Geometry check sheet. Reference: the model listing, model coordinates, mm. A direction names the side the tool comes from. Give positions to 0.01 mm unless a question says otherwise; leave off trailing zeros. Order: outer loops, then holes, each group sorted by start corner. A loop starts at its lowest first (then second) coordinate and runs counter-clockwise, first axis right, second up.
```python
from build123d import *

# Parameters (mm, degrees)
SKETCH1_W            = 100
SKETCH1_H            = 85
SKETCH1_W_2          = 80
SKETCH1_H_2          = 65
BOSS_EXTRUDE1_DEPTH  = 40
SKETCH14_W           = 5
SKETCH14_H           = 5
CUT_EXTRUDE11_DEPTH  = 10
CUT_EXTRUDE16_REACH  = 117.785
SKETCH24_W           = 22
SKETCH24_H           = 22
BOSS_EXTRUDE13_DEPTH = 6
CUT_EXTRUDE17_REACH  = 108.419
SKETCH32_W           = 22
SKETCH32_H           = 22
BOSS_EXTRUDE17_DEPTH = 6
SKETCH33_W           = 5
SKETCH33_H           = 5
CUT_EXTRUDE18_DEPTH  = 10
SKETCH36_W           = 22
SKETCH36_H           = 22
BOSS_EXTRUDE19_DEPTH = 5


with BuildPart() as part:
    # Sketch1 → Boss-Extrude1 (new body)
    with BuildSketch(Plane(origin=(0, 0, 0), x_dir=(0, 1, 0), z_dir=(0, 0, 1))):
        Rectangle(SKETCH1_W, SKETCH1_H)
        Rectangle(SKETCH1_W_2, SKETCH1_H_2, mode=Mode.SUBTRACT)
    extrude(amount=BOSS_EXTRUDE1_DEPTH)

    # Sketch14 → Cut-Extrude11 (cut)
    with BuildSketch(Plane.XY.offset(40)):
        with Locations((-37.671132401, 44.6965107)):
            Rectangle(SKETCH14_W, SKETCH14_H)
        with Locations((-37.671132401, -44.6965107)):
            Rectangle(SKETCH14_W, SKETCH14_H)
        with Locations((37.671132401, 44.6965107)):
            Rectangle(SKETCH14_W, SKETCH14_H)
        with Locations((37.671132401, -44.6965107)):
            Rectangle(SKETCH14_W, SKETCH14_H)
        with Locations((0, 44.6965107)):
            Rectangle(SKETCH14_W, SKETCH14_H)
        with Locations((0, -44.6965107)):
            Rectangle(SKETCH14_W, SKETCH14_H)
        with Locations((-37.671132401, 0)):
            Rectangle(SKETCH14_W, SKETCH14_H)
    extrude(amount=-CUT_EXTRUDE11_DEPTH, mode=Mode.SUBTRACT)

    # Sketch22 → Cut-Extrude16 (cut, up to next)
    with BuildSketch(Plane(origin=(0, 50, 0), x_dir=(-1, 0, 0), z_dir=(0, 1, 0)), mode=Mode.PRIVATE) as cut_extrude16_sk1:
        with BuildLine():
            Line((-6, 9.521249719), (6, 9.521249719))
            ThreePointArc((6, 9.521249719), (10, 5.521249719), (6, 1.521249719))
            Line((6, 1.521249719), (-6, 1.521249719))
            ThreePointArc((-6, 1.521249719), (-10, 5.521249719), (-6, 9.521249719))
        make_face()
    cut_extrude16_tool1 = extrude(cut_extrude16_sk1.sketch, amount=-CUT_EXTRUDE16_REACH, mode=Mode.PRIVATE) & part.part
    add(cut_extrude16_tool1.solids().sort_by_distance((0, 50, 5.52125))[0], mode=Mode.SUBTRACT)

    # Sketch24 → Boss-Extrude13 (add)
    with BuildSketch(Plane.XY.offset(16)):
        with Locations((21.5, 2.716540801)):
            Rectangle(SKETCH24_W, SKETCH24_H)
    extrude(amount=BOSS_EXTRUDE13_DEPTH)

    # Sketch12 → Cut-Extrude17 (cut, up to next)
    with BuildSketch(Plane.YZ.offset(42.5), mode=Mode.PRIVATE) as cut_extrude17_sk1:
        with BuildLine():
            Line((-17.870386686, 34.517617013), (17.870386686, 34.517617013))
            ThreePointArc((17.870386686, 34.517617013), (19.229729644, 33.158274056), (17.870386686, 31.798931098))
            Line((17.870386686, 31.798931098), (-17.870386686, 31.798931098))
            ThreePointArc((-17.870386686, 31.798931098), (-19.229729644, 33.158274056), (-17.870386686, 34.517617013))
        make_face()
    cut_extrude17_tool1 = extrude(cut_extrude17_sk1.sketch, amount=-CUT_EXTRUDE17_REACH, mode=Mode.PRIVATE) & part.part
    # Sketch12 → Cut-Extrude17 (cut, up to next)
    with BuildSketch(Plane.YZ.offset(42.5), mode=Mode.PRIVATE) as cut_extrude17_sk2:
        with BuildLine():
            Line((-17.870386686, 29.316472465), (17.870386686, 29.316472465))
            ThreePointArc((17.870386686, 29.316472465), (19.31261641, 27.874242742), (17.870386686, 26.432013019))
            Line((17.870386686, 26.432013019), (-17.870386686, 26.432013019))
            ThreePointArc((-17.870386686, 26.432013019), (-19.31261641, 27.874242742), (-17.870386686, 29.316472465))
        make_face()
    cut_extrude17_tool2 = extrude(cut_extrude17_sk2.sketch, amount=-CUT_EXTRUDE17_REACH, mode=Mode.PRIVATE) & part.part
    add(cut_extrude17_tool1.solids().sort_by_distance((42.5, 0, 33.158274))[0], mode=Mode.SUBTRACT)
    add(cut_extrude17_tool2.solids().sort_by_distance((42.5, 0, 27.874243))[0], mode=Mode.SUBTRACT)

    # Sketch32 → Boss-Extrude17 (add)
    with BuildSketch(Plane.XY.offset(16)):
        with Locations((-2.810397874, 29)):
            Rectangle(SKETCH32_W, SKETCH32_H)
    extrude(amount=BOSS_EXTRUDE17_DEPTH)

    # Sketch33 → Cut-Extrude18 (cut)
    with BuildSketch(Plane(origin=(0, 0, 0), x_dir=(1, 0, 0), z_dir=(0, 0, -1))):
        with Locations((-37.671132401, 44.6965107)):
            Rectangle(SKETCH33_W, SKETCH33_H)
        with Locations((0, 44.6965107)):
            Rectangle(SKETCH33_W, SKETCH33_H)
        with Locations((37.671132401, 44.6965107)):
            Rectangle(SKETCH33_W, SKETCH33_H)
        with Locations((-37.671132401, 0)):
            Rectangle(SKETCH33_W, SKETCH33_H)
        with Locations((-37.671132401, -44.6965107)):
            Rectangle(SKETCH33_W, SKETCH33_H)
        with Locations((37.671132401, -44.6965107)):
            Rectangle(SKETCH33_W, SKETCH33_H)
    extrude(amount=-CUT_EXTRUDE18_DEPTH, mode=Mode.SUBTRACT)

    # Sketch36 → Boss-Extrude19 (add)
    with BuildSketch(Plane.XY.offset(23)):
        with Locations((-21.5, 3.296429393)):
            Rectangle(SKETCH36_W, SKETCH36_H)
    extrude(amount=BOSS_EXTRUDE19_DEPTH)


solid = part.part
```
Q1. Access from +Z, -Z, +X, -X, +Y, -Y to the whole of each face (thin tool, end or side, straight path). Record for faces 1 (the face through (-38, -45, 30)), 2 (the face through (38, 0, 34.518)), 3 (the face through (-40.171, 45, 5)), 4 (the face through (-13.81, 29, 19)).
Q2. Gauge pin test, flat ends, axial feed: P1, Ø2, axis at x = -24, y = 1, coming from the -Z side; P2, Ø6, axis at x = -30, y = 18.5, coming from the -Z side; P3, Ø11, axis at x = -19.5, y = 2, coming from the +Z side. Record the tip position at first contact, or that the pin passes through.
Q3. Cross-section at C-C, the plane y = -16. Record the boundary of the cut face in (x, z).
Q4. Cross-section at D-D, the plane y = 43.5. Record the boundary of the cut face in (x, z).
Q5. Cross-section at B-B, the plane y = -26.5. Record the boundary of the cut face in (x, z).
Q6. Release check for a two-part mould opening along Y. For faces 5 (the face through (21, 3, 22)), 6 (the face through (42.5, -1, 20)) record: pulls with the +Y half, pulls with the -Y half, needs draft (parallel to the pull), parting line crosses it, or undercut.
Q7. Thickness scan on L1, parallel to Y at x = 36, z = 38.5; L2, parallel to X at y = 24.5, z = 20; L3, parallel to Y at x = -36, z = 35. Record the ranges inside material, lowest first.
Q8. Cross-section at A-A, the plane x = 13. Record the boundary of the cut face in (y, z).
Answers follow:
1. face 1: +Z
1. face 2: +X
1. face 3: -Z
1. face 4: +Z, -Z
2. P1: stops at z = 23
2. P2: stops at z = 0
2. P3: stops at z = 28
3. outline: (-42.5, 0) - (-32.5, 0) - (-32.5, 40) - (-42.5, 40) - close; (32.5, 0) - (42.5, 0) - (42.5, 26.43) - (32.5, 26.43) - close; (32.5, 29.32) - (42.5, 29.32) - (42.5, 31.8) - (32.5, 31.8) - close; (32.5, 34.52) - (42.5, 34.52) - (42.5, 40) - (32.5, 40) - close
4. outline: (-42.5, 0) - (-40.17, 0) - (-40.17, 10) - (-35.17, 10) - (-35.17, 0) - (35.17, 0) - (35.17, 10) - (40.17, 10) - (40.17, 0) - (42.5, 0) - (42.5, 40) - (40.17, 40) - (40.17, 30) - (35.17, 30) - (35.17, 40) - (2.5, 40) - (2.5, 30) - (-2.5, 30) - (-2.5, 40) - (-35.17, 40) - (-35.17, 30) - (-40.17, 30) - (-40.17, 40) - (-42.5, 40) - close; hole (-6, 1.52) - (6, 1.52) arc R4 ccw to (6, 9.52) - (-6, 9.52) arc R4 ccw to start
5. outline: (-42.5, 0) - (-32.5, 0) - (-32.5, 40) - (-42.5, 40) - close; (32.5, 0) - (42.5, 0) - (42.5, 40) - (32.5, 40) - close
6. face 5: undercut
6. face 6: needs draft
7. L1: y = -50 to -47.2, -42.2 to 42.2, 47.2 to 50
7. L2: x = -42.5 to -32.5, -13.81 to 8.19, 32.5 to 42.5
7. L3: y = -50 to -47.2, -42.2 to -2.5, 2.5 to 42.2, 47.2 to 50
8. outline: (-50, 0) - (-40, 0) - (-40, 40) - (-50, 40) - close; (-8.28, 16) - (13.72, 16) - (13.72, 22) - (-8.28, 22) - close; (40, 0) - (50, 0) - (50, 40) - (40, 40) - close
